For this review, take the finished solid that the model builds, in its own axes (mm). Round coordinates to 2 decimals unless told otherwise and drop trailing zeros. Order: outer loops, then holes, each group sorted by start corner. A loop starts at its lowest first (then second) coordinate and runs counter-clockwise, first axis right, second up. Notation, with made-up numbers: (81.25, -31.75) -> (85.25, -31.75) arc R22 cw to (85.25, 5.25) -> close; hole circle Ø6 at (3.25, 34). An arc over 180 degrees is marked (long way). Answer in a Markdown table with one row per item.
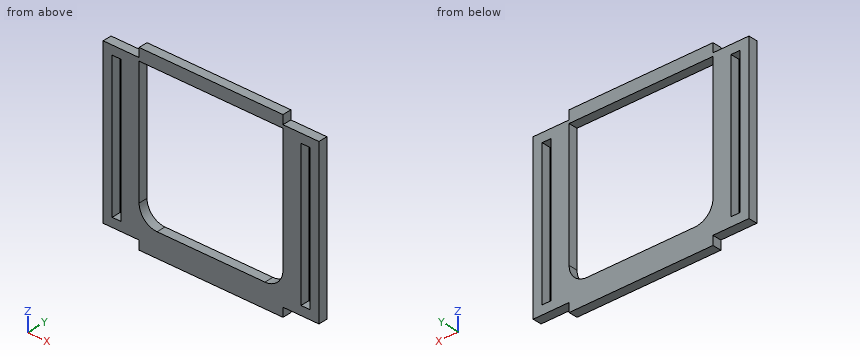
```python
from build123d import *

# Parameters (mm, degrees)
SKETCH1_W               = 152.4
SKETCH1_H               = 127
BOSS_EXTRUDE1_DEPTH     = 6.35
SKETCH2_W               = 25.4
SKETCH2_H               = 6.35
SKETCH2_W_2             = 6.35
SKETCH2_H_2             = 101.6
CUT_EXTRUDE1_DEPTH      = 7.35
CUT_EXTRUDE1_DEPTH_BACK = 6.35
CUT_EXTRUDE2_DEPTH      = 127
CUT_EXTRUDE2_DEPTH_BACK = 127


with BuildPart() as part:
    # Sketch1 → Boss-Extrude1 (new body)
    with BuildSketch(Plane(origin=(0, 0, 0), x_dir=(1, 0, 0), z_dir=(0, 1, 0))):
        Rectangle(SKETCH1_W, SKETCH1_H)
    extrude(amount=BOSS_EXTRUDE1_DEPTH)

    # Sketch2 → Cut-Extrude1 (cut, two sides)
    with BuildSketch(Plane(origin=(0, 0, 0), x_dir=(1, 0, 0), z_dir=(0, 1, 0))) as cut_extrude1_sk:
        with Locations((-63.5, 60.325)):
            Rectangle(SKETCH2_W, SKETCH2_H)
        with Locations((-63.5, -60.325)):
            Rectangle(SKETCH2_W, SKETCH2_H)
        with Locations((63.5, -60.325)):
            Rectangle(SKETCH2_W, SKETCH2_H)
        with Locations((63.5, 60.325)):
            Rectangle(SKETCH2_W, SKETCH2_H)
        with Locations((66.675, 0)):
            Rectangle(SKETCH2_W_2, SKETCH2_H_2)
        with Locations((-66.675, 0)):
            Rectangle(SKETCH2_W_2, SKETCH2_H_2)
    extrude(amount=CUT_EXTRUDE1_DEPTH, mode=Mode.SUBTRACT)
    extrude(cut_extrude1_sk.sketch, amount=-CUT_EXTRUDE1_DEPTH_BACK, mode=Mode.SUBTRACT)

    # Sketch3 → Cut-Extrude2 (cut, two sides)
    with BuildSketch(Plane(origin=(0, 0, 0), x_dir=(1, 0, 0), z_dir=(0, 1, 0))) as cut_extrude2_sk:
        with BuildLine():
            Line((-50.8, -54.914183245), (50.8, -54.914183245))
            Line((50.8, -54.914183245), (50.8, 33.985816755))
            ThreePointArc((50.8, 33.985816755), (47.080256121, 42.966072876), (38.1, 46.685816755))
            Line((38.1, 46.685816755), (-38.1, 46.685816755))
            ThreePointArc((-38.1, 46.685816755), (-47.080256121, 42.966072876), (-50.8, 33.985816755))
            Line((-50.8, 33.985816755), (-50.8, -54.914183245))
        make_face()
    extrude(amount=CUT_EXTRUDE2_DEPTH, mode=Mode.SUBTRACT)
    extrude(cut_extrude2_sk.sketch, amount=-CUT_EXTRUDE2_DEPTH_BACK, mode=Mode.SUBTRACT)


solid = part.part
```
Q1. Take a section at A-A, the plane x = -1. Write out the cut boundary in (y, z).
Answer key:
| item | result |
|---|---|
| outline | (0, -63.5) -> (6.35, -63.5) -> (6.35, -46.69) -> (0, -46.69) -> close; (0, 54.91) -> (6.35, 54.91) -> (6.35, 63.5) -> (0, 63.5) -> close |
Q2. Take a section at C-C, the plane y = 1.5. Write out the cut boundary in (x, z), then the cut area to 3 significant figures.
Answer key:
| item | result |
|---|---|
| outline | (-76.2, -57.15) -> (-50.8, -57.15) -> (-50.8, -63.5) -> (50.8, -63.5) -> (50.8, -57.15) -> (76.2, -57.15) -> (76.2, 57.15) -> (50.8, 57.15) -> (50.8, 63.5) -> (-50.8, 63.5) -> (-50.8, 57.15) -> (-76.2, 57.15) -> close; hole (-69.85, -50.8) -> (-63.5, -50.8) -> (-63.5, 50.8) -> (-69.85, 50.8) -> close; hole (-50.8, -33.99) arc R12.7 ccw to (-38.1, -46.69) -> (38.1, -46.69) arc R12.7 ccw to (50.8, -33.99) -> (50.8, 54.91) -> (-50.8, 54.91) -> close; hole (63.5, -50.8) -> (69.85, -50.8) -> (69.85, 50.8) -> (63.5, 50.8) -> close |
| area | 7,170 mm^2 |
Q3. Take a section at B-B, the plane z = 49. Write out the cut boundary in (x, y).
Answer key:
| item | result |
|---|---|
| outline | (-76.2, 0) -> (-69.85, 0) -> (-69.85, 6.35) -> (-76.2, 6.35) -> close; (-63.5, 0) -> (-50.8, 0) -> (-50.8, 6.35) -> (-63.5, 6.35) -> close; (50.8, 0) -> (63.5, 0) -> (63.5, 6.35) -> (50.8, 6.35) -> close; (69.85, 0) -> (76.2, 0) -> (76.2, 6.35) -> (69.85, 6.35) -> close |
Q4. Clearance check with flat-ended pins moving along their axes: pin 1 Ø1.9 at (x, y) = (-59.5, 2) entering from -Z; pin 2 Ø1.9 at (y, z) = (2.5, 61.5) entering from -X. State where each tip first meets the part, or that it passes through.
Answer key:
| item | result |
|---|---|
| pin 1 | stops at z = -57.15 |
| pin 2 | stops at x = -50.8 |
Q5. To check wall thickness, follow probe 1 along X at (y, z) = (5.25, -34); probe 2 along Z at (x, y) = (-7, 2); probe 3 along X at (y, z) = (4.25, -45). State the ranges of each line that lie inside material, in increasing order.
Answer key:
| item | result |
|---|---|
| probe 1 | x = -76.2 to -69.85, -63.5 to -50.8, 50.8 to 63.5, 69.85 to 76.2 |
| probe 2 | z = -63.5 to -46.69, 54.91 to 63.5 |
| probe 3 | x = -76.2 to -69.85, -63.5 to -44.42, 44.42 to 63.5, 69.85 to 76.2 |
